from build123d import *

# Parameters (mm, degrees)
MODEL_W             = 5.5
MODEL_H             = 5.5
BOSS_EXTRUDE1_DEPTH = 6


with BuildPart() as part:
    # Model → Boss-Extrude1 (new body)
    with BuildSketch(Plane.XY):
        with BuildLine():
            Line((3385.437630562, 1476.840270732), (3395.437630562, 1476.840270732))
            Line((3395.437630562, 1476.840270732), (3406.437630562, 1476.840270732))
            Line((3406.437630562, 1476.840270732), (3406.437630562, 1504.786647956))
            ThreePointArc((3406.437630562, 1504.786647956), (3436.437630562, 1517.840270732), (3466.437630562, 1504.786647956))
            Line((3466.437630562, 1504.786647956), (3466.437630562, 1476.840270732))
            Line((3466.437630562, 1476.840270732), (3468.937630562, 1476.840270732))
            Line((3468.937630562, 1476.840270732), (3468.937630562, 1470.840270732))
            Line((3468.937630562, 1470.840270732), (3474.937630562, 1470.840270732))
            Line((3474.937630562, 1470.840270732), (3474.937630562, 1476.840270732))
            Line((3474.937630562, 1476.840270732), (3487.437630562, 1476.840270732))
            ThreePointArc((3487.437630562, 1476.840270732), (3436.437630562, 1527.840270732), (3385.437630562, 1476.840270732))
        make_face()
        with Locations((3471.937630562, 1482.340270732)):
            Rectangle(MODEL_W, MODEL_H, mode=Mode.SUBTRACT)
        with Locations((3471.937630562, 1502.340270732)):
            Rectangle(MODEL_W, MODEL_H, mode=Mode.SUBTRACT)
        with Locations((3400.937630562, 1482.340270732)):
            Rectangle(MODEL_W, MODEL_H, mode=Mode.SUBTRACT)
        with Locations((3400.937630562, 1502.340270732)):
            Rectangle(MODEL_W, MODEL_H, mode=Mode.SUBTRACT)
    extrude(amount=BOSS_EXTRUDE1_DEPTH)


solid = part.part
Could you check a few things on this model? Use its own coordinates, in mm. A direction names the side the tool comes from. Round coordinates to 2 decimals unless told otherwise and drop trailing zeros. Order: outer loops, then holes, each group sorted by start corner. A loop starts at its lowest first (then second) coordinate and runs counter-clockwise, first axis right, second up.
Q1. Please list where these lines run through material, in increasing order: probe 1 along X at (y, z) = (1504, 1); probe 2 along X at (y, z) = (1485, 0.7); probe 3 along X at (y, z) = (1477, 4.5).
Geometry says:
probe 1: x = 3393.27 to 3398.19, 3403.69 to 3406.44, 3466.44 to 3469.19, 3474.69 to 3479.6
probe 2: x = 3386.09 to 3398.19, 3403.69 to 3406.44, 3466.44 to 3469.19, 3474.69 to 3486.78
probe 3: x = 3385.44 to 3406.44, 3466.44 to 3487.44
Q2. Which directions (+Z, -Z, +X, -X, +Y, -Y) give clear straight access to the entire face, cutting with the end or side of a thin tool? Please do faces 1 (the face through (3436, 1518, 6)), 2 (the face through (3436, 1518, 0)), 3 (the face through (3466.438, 1491, 3)), 4 (the face through (3468, 1476.84, 3)), 5 (the face through (3469.188, 1502, 3)).
Geometry says:
face 1: +Z, +X, -X, +Y, -Y
face 2: -Z, +X, -X, +Y, -Y
face 3: +Z, -Z, -Y
face 4: +Z, -Z, -X, -Y
face 5: +Z, -Z
Q3. Imagine slicing it at C-C, the plane x = 3472. List the corners of the cut face in (y, z) for me.
Geometry says:
outline: (1470.84, 0) - (1479.59, 0) - (1479.59, 6) - (1470.84, 6) - close; (1485.09, 0) - (1499.59, 0) - (1499.59, 6) - (1485.09, 6) - close; (1505.09, 0) - (1513.4, 0) - (1513.4, 6) - (1505.09, 6) - close
Q4. Imagine slicing it at B-B, the plane y = 1491. List the corners of the cut face in (x, z) for me, then the cut area to 3 significant figures.
Geometry says:
outline: (3387.44, 0) - (3406.44, 0) - (3406.44, 6) - (3387.44, 6) - close; (3466.44, 0) - (3485.43, 0) - (3485.43, 6) - (3466.44, 6) - close
area: 228 mm2
Q5. I'm going to push flat-ended pins straight in: P1, Ø1.6, axis at x = 3399.5, z = 2, coming from the +Y side; P2, Ø1.5, axis at y = 1516.5, z = 3, coming from the -X side; P3, Ø3, axis at y = 1502.5, z = 4.5, coming from the -X side. Where does each tip first touch, or does it pass through?
Geometry says:
P1: stops at y = 1512.83
P2: stops at x = 3403.47
P3: stops at x = 3391.52
Q6. Thinking about a two-plate mould opening in X: for faces 6 (the face through (3481, 1476.84, 3)), 7 (the face through (3474.938, 1474, 3)), 8 (the face through (3472, 1505.09, 3)), which applies, released by +X, released by -X, zero draft, split by the parting line, or undercut?
Geometry says:
face 6: zero draft
face 7: released by +X
face 8: undercut
Q7. Imagine slicing it at D-D, the plane y = 1513. List the corners of the cut face in (x, z) for me, then the cut area to 3 significant figures.
Geometry says:
outline: (3400.47, 0) - (3417.11, 0) - (3417.11, 6) - (3400.47, 6) - close; (3455.76, 0) - (3472.4, 0) - (3472.4, 6) - (3455.76, 6) - close
area: 200 mm2
Q8. Imagine slicing it at A-A, the plane z = 0.95. List the corners of the cut face in (x, y) for me.
Geometry says:
outline: (3385.44, 1476.84) - (3406.44, 1476.84) - (3406.44, 1504.79) arc R41 cw to (3466.44, 1504.79) - (3466.44, 1476.84) - (3468.94, 1476.84) - (3468.94, 1470.84) - (3474.94, 1470.84) - (3474.94, 1476.84) - (3487.44, 1476.84) arc R51 ccw to start; hole (3398.19, 1479.59) - (3403.69, 1479.59) - (3403.69, 1485.09) - (3398.19, 1485.09) - close; hole (3398.19, 1499.59) - (3403.69, 1499.59) - (3403.69, 1505.09) - (3398.19, 1505.09) - close; hole (3469.19, 1479.59) - (3474.69, 1479.59) - (3474.69, 1485.09) - (3469.19, 1485.09) - close; hole (3469.19, 1499.59) - (3474.69, 1499.59) - (3474.69, 1505.09) - (3469.19, 1505.09) - close
